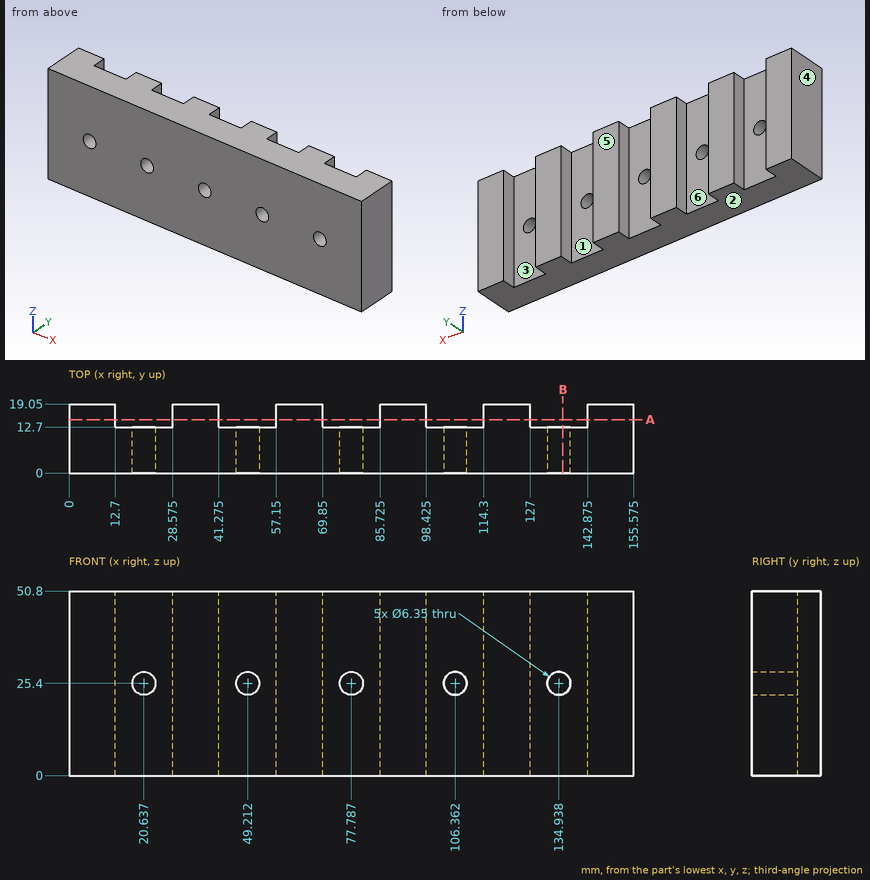
Can you work these out from the drawing? Everything is in mm from the part's minimum corner. A direction names the side the tool comes from. Round coordinates to 2 decimals unless told otherwise and drop trailing zeros. Write each loop counter-clockwise with the first axis right and the second up, starting at its lowest first coordinate (ties: lowest second). Pieces come first, ordered by that corner, then holes.
1. For the marked faces 1 and 2, which set-ups out of +Z, -Z, +X, -X, +Y, -Y let a thin tool reach every point of the face, with its end or its side?
2. I need wall thicknesses on L1, parallel to X at y = 3.75, z = 25.4 (1 decimal); L2, parallel to Z at x = 133.5, y = 12; L3, parallel to X at y = 10.75, z = 23 (1 decimal). Which ranges of each line are inside material? Lowest first, please.
3. Suppose I cut it at B-B (x = 136). List the corners of the cut face in (y, z) for me.
4. If we mould it in two halves opening along X, with no side actions, what happens to the marked faces 3, 4, 5 and 6? For each: released by +X, released by -X, zero draft, split by the parting line, or undercut.
5. Will these pins go through, and if not, where does the flat tip stop? pin 1 Ø17.5 at (x, z) = (78, 27) entering from +Y; pin 2 Ø5 at (x, z) = (133, 29) entering from +Y.
6. Suppose I cut it at A-A (y = 14.75). State how many separate pieces and enclosed holes the cut face has, and give its area (3 significant figures).
Answer sheet:
1. face 1: +Z, -Z, +Y
1. face 2: -Z, +X, -X, +Y, -Y
2. L1: x = 0 to 17.5, 23.8 to 46, 52.4 to 74.6, 81 to 103.2, 109.5 to 131.8, 138.1 to 155.6
2. L2: z = 0 to 22.57, 28.23 to 50.8
2. L3: x = 0 to 18.6, 22.7 to 47.1, 51.3 to 75.7, 79.9 to 104.3, 108.4 to 132.9, 137 to 155.6
3. outline: (0, 0) - (12.7, 0) - (12.7, 22.41) - (0, 22.41) - close; (0, 28.39) - (12.7, 28.39) - (12.7, 50.8) - (0, 50.8) - close
4. face 3: undercut
4. face 4: released by -X
4. face 5: zero draft
4. face 6: undercut
5. pin 1: stops at y = 19.05
5. pin 2: stops at y = 12.7
6. separate pieces: 6
6. enclosed holes: 0
6. area: 3,870 mm2
